from build123d import *

# Parameters (mm, degrees)
SKETCH001_R  = 2.5
PAD001_DEPTH = 30
SKETCH_R     = 9.25
PAD_DEPTH    = 15


with BuildPart() as pad001:
    # Sketch001 → Pad001 (new body)
    with BuildSketch(Plane.XY):
        Circle(SKETCH001_R)
    extrude(amount=PAD001_DEPTH)


with BuildPart() as fusion:
    # Sketch → Pad (new body)
    with BuildSketch(Plane.XY):
        Circle(SKETCH_R)
    extrude(amount=PAD_DEPTH)

    # Fusion: union Pad001
    add(pad001.part)


solid = fusion.part
Input: part model. Units: mm. Frame: model coordinates. A direction names the side the tool comes from. Give positions to 0.01 mm unless a question says otherwise; leave off trailing zeros. Order: outer loops, then holes, each group sorted by start corner. A loop starts at its lowest first (then second) coordinate and runs counter-clockwise, first axis right, second up. Notation, with made-up numbers: (25.25, -38.5) -> (34.25, -38.5) arc R29 cw to (34.25, -5.5) -> close; hole circle Ø8 at (23, 89.5). An arc over 180 degrees is marked (long way). Use one line per item in the form item = value.
1) Section C-C, the plane z = 11.5. Return loops of the section in (x, y).
Response values:
outline = circle Ø18.5 at (0, 0)
2) Section A-A, the plane y = 0. Return loops of the section in (x, z).
Response values:
outline = (-9.25, 0) -> (9.25, 0) -> (9.25, 15) -> (2.5, 15) -> (2.5, 30) -> (-2.5, 30) -> (-2.5, 15) -> (-9.25, 15) -> close
3) Line query: probe 1 along Z at (x, y) = (-8, -3.25); probe 2 along X at (y, z) = (-0.25, 11.5); probe 3 along Y at (x, z) = (5.5, 12.75). Output: solid intervals per line, ascending.
Response values:
probe_1 = 0 to 15
probe_2 = -9.25 to 9.25
probe_3 = -7.44 to 7.44
4) First-contact query: pin 1 Ø5 at (x, z) = (0, 26.5) entering from -Y; pin 2 Ø1.5 at (x, z) = (1.5, 20.5) entering from +Y; pin 3 Ø8 at (x, z) = (-6.5, 11.5) entering from +Y. Flat tips, straight axial feed; report the tip coordinate or a pass-through.
Response values:
pin_1 = -2.5
pin_2 = 2.38
pin_3 = 8.91
5) Reachability of faces 1 (the cylindrical face through (-2.01, -9.03, 7.4)), 2 (the cylindrical face through (-0.54, -2.44, 22.4)) from +Z, -Z, +X, -X, +Y, -Y: full face, straight path, thin tool, end or side. Return the list, or none.
Response values:
face_1 = +Z, -Z
face_2 = +Z
6) Section D-D, the plane z = 26.25. Return loops of the section in (x, y), and give its area (3 significant figures).
Response values:
outline = circle Ø5 at (0, 0)
area = 19.6 mm^2
